Design review of the part built by this model. Coordinates are the model's own, in mm. Face numbers are marked on the shaded views. Give positions to 0.01 mm unless a question says otherwise; leave off trailing zeros. Order: outer loops, then holes, each group sorted by start corner. A loop starts at its lowest first (then second) coordinate and runs counter-clockwise, first axis right, second up. Notation, with made-up numbers: (-29, 25) -> (-14, 25) arc R31 ccw to (-14, 59) -> close; hole circle Ø9 at (53, 22). An arc over 180 degrees is marked (long way). One line per item, written item: value. Start each with the question number.
1) The part is to be moulded in two halves that separate along X. For the marked faces 1, 2 and 3, say which applies: released by +X, released by -X, zero draft, split by the parting line, or undercut.
2) Consider section B-B (z = 0). State the section outline as (x, y) points, plus the area to 3 significant figures.
3) For pin 1 (3 mm diameter, centred on y = 15.5, z = 2, fed in from -X); pin 2 (10 mm diameter, centred on x = 24.5, z = 12.5, fed in from -Y); pin 3 (12 mm diameter, centred on x = -23, y = 12.5, fed in from +Z), all flat-tipped, find the tip position at first contact; note any pin that passes through.
4) Wall thickness on line 1 along X through (y, z) = (13.75, 0); line 2 along X through (y, z) = (5, 0); line 3 along Y through (x, z) = (-25.5, 17.5): over which ranges is each line inside the solid? List them lowest first. Write a range as from..to.
5) Consider section A-A (x = 0). State the section outline as (y, z) points.
6) Consider section D-D (x = -8). State the section outline as (y, z) points.
7) Consider section C-C (y = 8). State the section outline as (x, z) points.
from build123d import *

# Parameters (mm, degrees)
SKETCH1_R          = 14.986
BASE_DEPTH         = 10.16
SKETCH2_R          = 31.496
GEAR_DEPTH         = 11.938
SKETCH3_R          = 6
CUT_EXTRUDE1_DEPTH = 50.722405774


with BuildPart() as part:
    # Sketch1 → Base (new body)
    with BuildSketch(Plane(origin=(0, 0, 0), x_dir=(1, 0, 0), z_dir=(0, 1, 0))):
        with Locations(Location((0, 0, 0), (0, 0, 270))):
            Circle(SKETCH1_R)
    extrude(amount=BASE_DEPTH)

    # Sketch2 → Gear (add)
    with BuildSketch(Plane(origin=(0, 10.16, 0), x_dir=(1, 0, 0), z_dir=(0, 1, 0))):
        with Locations(Location((0, 0, 0), (0, 0, 270))):
            Circle(SKETCH2_R)
    extrude(amount=GEAR_DEPTH)

    # Sketch3 → Cut-Extrude1 (cut, through all)
    with BuildSketch(Plane(origin=(0, 22.098, 0), x_dir=(1, 0, 0), z_dir=(0, 1, 0))):
        with Locations(Location((0, 0, 0), (0, 0, 270))):
            Circle(SKETCH3_R)
    extrude(amount=-CUT_EXTRUDE1_DEPTH, mode=Mode.SUBTRACT)


solid = part.part
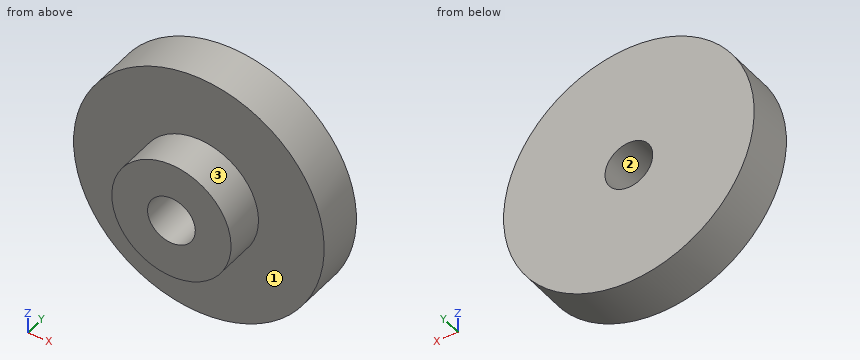
Checked values:
1. face 1: zero draft
1. face 2: undercut
1. face 3: split by the parting line
2. outline: (-31.5, 10.16) -> (-14.99, 10.16) -> (-14.99, 0) -> (-6, 0) -> (-6, 22.1) -> (-31.5, 22.1) -> close; (6, 0) -> (14.99, 0) -> (14.99, 10.16) -> (31.5, 10.16) -> (31.5, 22.1) -> (6, 22.1) -> close
2. area: 791 mm^2
3. pin 1: stops at x = -31.49
3. pin 2: stops at y = 10.16
3. pin 3: stops at z = 26.51
4. line 1: x = -31.5..-6, 6..31.5
4. line 2: x = -14.99..-6, 6..14.99
4. line 3: y = 10.16..22.1
5. outline: (0, -14.99) -> (10.16, -14.99) -> (10.16, -31.5) -> (22.1, -31.5) -> (22.1, -6) -> (0, -6) -> close; (0, 6) -> (22.1, 6) -> (22.1, 31.5) -> (10.16, 31.5) -> (10.16, 14.99) -> (0, 14.99) -> close
6. outline: (0, -12.67) -> (10.16, -12.67) -> (10.16, -30.46) -> (22.1, -30.46) -> (22.1, 30.46) -> (10.16, 30.46) -> (10.16, 12.67) -> (0, 12.67) -> close
7. outline: circle Ø29.97 at (0, 0); hole circle Ø12 at (0, 0)
